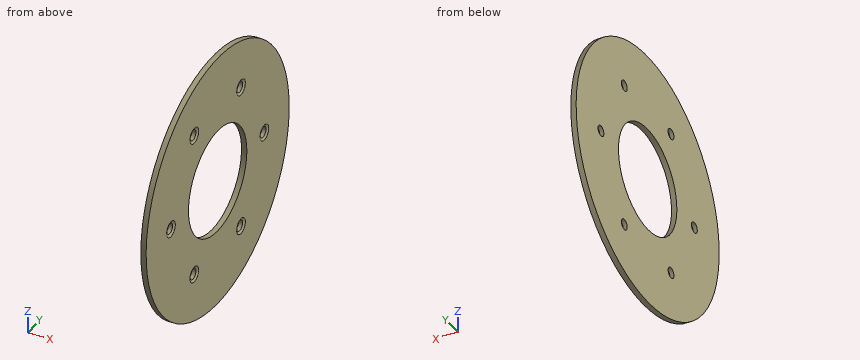
```python
from build123d import *

# Parameters (mm, degrees)
SKETCH1_R           = 49
SKETCH1_R_2         = 20
BOSS_EXTRUDE1_DEPTH = 2
SKETCH1_3_R         = 2
CUT_EXTRUDE2_DEPTH  = 0.5
SKETCH1_4_R         = 2
CUT_EXTRUDE3_DEPTH  = 70.32532005
CIRPATTERN1_COUNT   = 6
CIRPATTERN2_COUNT   = 6


with BuildPart() as part:
    # Sketch1 → Boss-Extrude1 (new body)
    with BuildSketch(Plane.YZ):
        with Locations(Location((0, 0, 0), (0, 0, 270))):
            Circle(SKETCH1_R)
        with Locations(Location((0, 0, 0), (0, 0, 270))):
            Circle(SKETCH1_R_2, mode=Mode.SUBTRACT)
    extrude(amount=BOSS_EXTRUDE1_DEPTH)

    # Sketch1_3 → Cut-Extrude2 (cut)
    with BuildSketch(Plane.YZ):
        with Locations(Location((32, 0, 0), (0, 0, 270))):
            Circle(SKETCH1_3_R)
    cut_extrude2 = extrude(amount=CUT_EXTRUDE2_DEPTH, mode=Mode.SUBTRACT)

    # Sketch1_4 → Cut-Extrude3 (cut, through all)
    with BuildSketch(Plane.YZ):
        with Locations(Location((32, 0, 0), (0, 0, 270))):
            Circle(SKETCH1_4_R)
    cut_extrude3 = extrude(amount=CUT_EXTRUDE3_DEPTH, mode=Mode.SUBTRACT)

    # CirPattern1: Cut-Extrude2, Cut-Extrude3 ×6 about axis
    cirpattern1_axis = Axis((0, 0, 0), (1, 0, 0))
    add([cut_extrude2.rotate(cirpattern1_axis, i * 360 / CIRPATTERN1_COUNT) for i in range(1, CIRPATTERN1_COUNT)], mode=Mode.SUBTRACT)
    add([cut_extrude3.rotate(cirpattern1_axis, i * 360 / CIRPATTERN1_COUNT) for i in range(1, CIRPATTERN1_COUNT)], mode=Mode.SUBTRACT)

    # Sketch3 → Cut-Revolve1 (revolve, cut)
    with BuildSketch(Plane(origin=(0, 16, 0), x_dir=(-1, 0, 0), z_dir=(0, 1, 0)), mode=Mode.PRIVATE) as cut_revolve1_sk:
        Polygon((-2.49931716, 31.685808566), (-2.49931716, 27.712812921), (-1.5, 27.712812921), (-1.5, 29.685860989), align=None)
    cut_revolve1 = revolve(cut_revolve1_sk.sketch.rotate(Axis((15.134577625, 16, 27.712812921), (-1, 0, 0)), 120), axis=Axis((15.134577625, 16, 27.712812921), (-1, 0, 0)), mode=Mode.SUBTRACT)

    # CirPattern2: Cut-Revolve1 ×6 about axis
    cirpattern2_axis = Axis((0, 0, 0), (1, 0, 0))
    for i in range(1, CIRPATTERN2_COUNT):
        add(cut_revolve1.rotate(cirpattern2_axis, i * 360 / CIRPATTERN2_COUNT), mode=Mode.SUBTRACT)


solid = part.part
```
Design review of the part built by this model. Coordinates are the model's own, in mm. Give positions to 0.01 mm unless a question says otherwise; leave off trailing zeros. Write each loop counter-clockwise with the first axis right and the second up, starting at its lowest first coordinate (ties: lowest second). Pieces come first, ordered by that corner, then holes.
(1) Add section C-C (y = -16). Give the boundary of the cut face in (x, z).
Checked values:
outline: (0, -46.31) - (2, -46.31) - (2, -30.69) - (1.51, -29.71) - (0, -29.71) - close; (0, -25.71) - (1.51, -25.71) - (2, -24.74) - (2, -12) - (0, -12) - close; (0, 12) - (2, 12) - (2, 24.74) - (1.51, 25.71) - (0, 25.71) - close; (0, 29.71) - (1.51, 29.71) - (2, 30.69) - (2, 46.31) - (0, 46.31) - close
(2) Add section B-B (y = 11.5). Give the boundary of the cut face in (x, z), and give its area (3 significant figures).
Checked values:
outline: (0, -47.63) - (2, -47.63) - (2, -16.36) - (0, -16.36) - close; (0, 16.36) - (2, 16.36) - (2, 47.63) - (0, 47.63) - close
area: 125 mm2
(3) Wall thickness on line 1 along Y through (x, z) = (1.3, 0); line 2 along Z through (x, y) = (0.4, 16); line 3 along Z through (x, y) = (0.5, -32): over which ranges is each line inside the solid? List them lowest first.
Checked values:
line 1: y = -49 to -34, -30 to -20, 20 to 30, 34 to 49
line 2: z = -46.31 to -29.71, -25.71 to -12, 12 to 25.71, 29.71 to 46.31
line 3: z = -37.11 to -2, 2 to 37.11
(4) Add section D-D (x = 0.85). Give the boundary of the cut face in (y, z), and give its area (3 significant figures).
Checked values:
outline: circle Ø98 at (0, 0); hole circle Ø4 at (-32, 0); hole circle Ø40 at (0, 0); hole circle Ø4 at (-16, -27.71); hole circle Ø4 at (-16, 27.71); hole circle Ø4 at (16, -27.71); hole circle Ø4 at (16, 27.71); hole circle Ø4 at (32, 0)
area: 6,210 mm2
(5) Add section A-A (z = 0). Give the boundary of the cut face in (x, y), and give its area (3 significant figures).
Checked values:
outline: (0, -49) - (2, -49) - (2, -34.97) - (1.51, -34) - (0, -34) - close; (0, -30) - (1.51, -30) - (2, -29.03) - (2, -20) - (0, -20) - close; (0, 20) - (2, 20) - (2, 29.03) - (1.51, 30) - (0, 30) - close; (0, 34) - (1.51, 34) - (2, 34.97) - (2, 49) - (0, 49) - close
area: 99.1 mm2
(6) Clearance check with a flat-ended pin moving along its axis: pin 1 Ø5 at (y, z) = (16, -27.71) entering from +X. State where the tip first meets the part, or that it passes through.
Checked values:
pin 1: stops at x = 1.76
